```python
from build123d import *

# Parameters (mm, degrees)
SKETCH1_W           = 63.5
SKETCH1_H           = 63.5
BOSS_EXTRUDE1_DEPTH = 76.2
SKETCH2_W           = 60.325
SKETCH2_H           = 60.325
CUT_EXTRUDE1_DEPTH  = 75.4
FILLET1_R           = 2.54
SKETCH3_R           = 3.175
CUT_EXTRUDE2_DEPTH  = 89.44526556
SKETCH4_R           = 4.064
CUT_EXTRUDE3_DEPTH  = 89.44526556


with BuildPart() as part:
    # Sketch1 → Boss-Extrude1 (new body)
    with BuildSketch(Plane.XY):
        Rectangle(SKETCH1_W, SKETCH1_H)
    extrude(amount=BOSS_EXTRUDE1_DEPTH)

    # Sketch2 → Cut-Extrude1 (cut)
    with BuildSketch(Plane.XY.offset(76.2)):
        Rectangle(SKETCH2_W, SKETCH2_H)
    extrude(amount=-CUT_EXTRUDE1_DEPTH, mode=Mode.SUBTRACT)

    # Fillet1
    fillet1_edges = [part.edges().sort_by_distance(p)[0] for p in [
        (31.75, -31.75, 38.1),
        (-31.75, -31.75, 38.1),
        (-31.75, 31.75, 38.1),
        (31.75, 31.75, 38.1),
    ]]
    fillet(fillet1_edges, radius=FILLET1_R)

    # Sketch3 → Cut-Extrude2 (cut, through all)
    with BuildSketch(Plane(origin=(0, 0, 0), x_dir=(-1, 0, 0), z_dir=(0, 0, -1))):
        with Locations((0, 19.05)):
            Circle(SKETCH3_R)
        with Locations((0, -19.05)):
            Circle(SKETCH3_R)
        Circle(SKETCH3_R)
        with Locations((19.05, 0)):
            Circle(SKETCH3_R)
        with Locations((-19.05, 0)):
            Circle(SKETCH3_R)
    extrude(amount=-CUT_EXTRUDE2_DEPTH, mode=Mode.SUBTRACT)

    # Sketch4 → Cut-Extrude3 (cut, through all)
    with BuildSketch(Plane(origin=(0, 0, 0), x_dir=(-1, 0, 0), z_dir=(0, 0, -1))):
        with Locations((-15.875, -19.05)):
            Circle(SKETCH4_R)
        with Locations((15.875, -19.05)):
            Circle(SKETCH4_R)
    extrude(amount=-CUT_EXTRUDE3_DEPTH, mode=Mode.SUBTRACT)


solid = part.part
```
Input: part model. Units: mm. Frame: model coordinates. A direction names the side the tool comes from. Give positions to 0.01 mm unless a question says otherwise; leave off trailing zeros. Loops run counter-clockwise (first coordinate to the right, second up) from the corner with the lowest first, then second, coordinate; pieces in that order, holes last.
1) Contact query for flat-ended pins moving along their axis: pin 1 (5 mm diameter, centred on x = 18, y = 21.5, fed in from +Z); pin 2 (6.5 mm diameter, centred on x = -15.875, y = -19.05, fed in from +Z). Output: stop coordinate, or through.
A:
pin 1: stops at z = 0.8
pin 2: passes through
2) Section query A-A on z = 29.5. Return the cut outline in (x, y), and give its area (3 significant figures).
A:
outline: (-31.75, -29.21) arc R2.54 ccw to (-29.21, -31.75) - (29.21, -31.75) arc R2.54 ccw to (31.75, -29.21) - (31.75, 29.21) arc R2.54 ccw to (29.21, 31.75) - (-29.21, 31.75) arc R2.54 ccw to (-31.75, 29.21) - close; hole (-30.16, -30.16) - (30.16, -30.16) - (30.16, 30.16) - (-30.16, 30.16) - close
area: 388 mm2
3) Line query: L1, parallel to X at y = 13, z = 10.5; L2, parallel to Y at x = 0, z = 0.45 (3 decimals). Output: solid intervals per line, ascending.
A:
L1: x = -31.75 to -30.16, 30.16 to 31.75
L2: y = -31.75 to -22.225, -15.875 to -3.175, 3.175 to 15.875, 22.225 to 31.75
4) Section query C-C on x = 17. Return the cut outline in (y, z).
A:
outline: (-31.75, 0) - (-22.96, 0) - (-22.96, 0.8) - (-30.16, 0.8) - (-30.16, 76.2) - (-31.75, 76.2) - close; (-15.14, 0) - (-2.42, 0) - (-2.42, 0.8) - (-15.14, 0.8) - close; (2.42, 0) - (31.75, 0) - (31.75, 76.2) - (30.16, 76.2) - (30.16, 0.8) - (2.42, 0.8) - close
5) Section query D-D on y = -19.05. Count the separate pieces of the cut face and the enclosed holes in it, and give its area (3 significant figures).
A:
separate pieces: 4
enclosed holes: 0
area: 272 mm2
6) Mould query, pull axis X, two halves, no side actions, for faces 1 (the flat face through (-31.75, 0, 38)), 2 (the flat face through (30.162, 0, 39)), 3 (the cylindrical face through (30.986, -31.026, 38.633)). Classes: released by +X, released by -X, zero draft, split by the parting line, or undercut.
A:
face 1: released by -X
face 2: undercut
face 3: released by +X
7) Reachability of faces 4 (the flat face through (0, -30.162, 39)), 5 (the cylindrical face through (0.69, -3.1, 0.39)) from +Z, -Z, +X, -X, +Y, -Y: full face, straight path, thin tool, end or side. Return the list, or none.
A:
face 4: +Z
face 5: +Z, -Z
